```python
from build123d import *

# Parameters (mm, degrees)
SKETCH1_W           = 12
SKETCH1_H           = 4
BOSS_EXTRUDE1_DEPTH = 8
SKETCH2_W           = 4
SKETCH2_H           = 12
BOSS_EXTRUDE2_DEPTH = 25
SKETCH3_W           = 7.5
SKETCH3_H           = 12
BOSS_EXTRUDE3_DEPTH = 4
CHAMFER1_SIZE       = 2
RIB1_REACH          = 35.425
SKETCH4_WALL_W      = 70.36529828
SKETCH4_WALL_H      = 12
RIB2_REACH          = 35.425
SKETCH5_WALL_W      = 70.36529828
SKETCH5_WALL_H      = 12
SKETCH7_R           = 1
CUT_EXTRUDE2_DEPTH  = 4
FILLET1_R           = 0.4


with BuildPart() as part:
    # Sketch1 → Boss-Extrude1 (new body)
    with BuildSketch(Plane(origin=(0, 0, 0), x_dir=(0, 0, -1), z_dir=(1, 0, 0))):
        with Locations((6, 2)):
            Rectangle(SKETCH1_W, SKETCH1_H)
    extrude(amount=BOSS_EXTRUDE1_DEPTH)

    # Sketch2 → Boss-Extrude2 (add)
    with BuildSketch(Plane.XZ):
        with Locations((6, -6)):
            Rectangle(SKETCH2_W, SKETCH2_H)
    extrude(amount=BOSS_EXTRUDE2_DEPTH)

    # Sketch3 → Boss-Extrude3 (add)
    with BuildSketch(Plane.XZ.offset(25)):
        with Locations((7.75, -6)):
            Rectangle(SKETCH3_W, SKETCH3_H)
    extrude(amount=BOSS_EXTRUDE3_DEPTH)

    # Chamfer1
    chamfer1_edges = [part.edges().sort_by_distance(p)[0] for p in [
        (8, 4, -6),
        (4, -29, -6),
    ]]
    chamfer(chamfer1_edges, length=CHAMFER1_SIZE)

    # Sketch4 wall → Rib1 (add, up to next)
    with BuildSketch(Plane(origin=(3.464466094, -0.535533906, -12), x_dir=(0.707106781187, -0.707106781187, 0), z_dir=(-0.707106781187, -0.707106781187, 0)), mode=Mode.PRIVATE) as rib1_sk1:
        with Locations((0, 6)):
            Rectangle(SKETCH4_WALL_W, SKETCH4_WALL_H)
    rib1_tool1 = extrude(rib1_sk1.sketch, amount=-RIB1_REACH, mode=Mode.PRIVATE) - part.part
    add(rib1_tool1.solids().sort_by_distance((3.464466094, -0.535533906, -12))[0])

    # Sketch5 wall → Rib2 (add, up to next)
    with BuildSketch(Plane(origin=(8.535533906, -24.464466094, 0), x_dir=(0.707106781187, -0.707106781187, 0), z_dir=(0.707106781187, 0.707106781187, 0)), mode=Mode.PRIVATE) as rib2_sk1:
        with Locations((0, 6)):
            Rectangle(SKETCH5_WALL_W, SKETCH5_WALL_H)
    rib2_tool1 = extrude(rib2_sk1.sketch, amount=-RIB2_REACH, mode=Mode.PRIVATE) - part.part
    add(rib2_tool1.solids().sort_by_distance((8.535533906, -24.464466094, 0))[0])

    # Sketch7 → Cut-Extrude2 (cut)
    with BuildSketch(Plane.ZY):
        with Locations((-6, 2)):
            Circle(SKETCH7_R)
    extrude(amount=-CUT_EXTRUDE2_DEPTH, mode=Mode.SUBTRACT)

    # Fillet1
    fillet1_edges = [part.edges().sort_by_distance(p)[0] for p in [
        (11.5, -25, -6),
        (11.5, -27, -12),
        (10.285533906, -25, 0),
        (11.5, -27, 0),
        (11.5, -29, -6),
        (8.75, -29, 0),
        (8.75, -29, -12),
        (6, -29, -6),
        (3, 4, -12),
        (4, -14.035533906, -12),
        (7, 3, -12),
        (5, -28, -12),
        (4, -14.035533906, 0),
        (4, -27, -6),
        (8, -10.964466094, 0),
        (3, 4, 0),
        (7, 3, 0),
        (5, -28, 0),
        (0, 4, -6),
        (8, 2, -6),
        (6, 4, -6),
        (0, 2, -12),
        (0, 0, -6),
        (4, -1.071067812, -6),
        (0, 2, 0),
        (1.464466094, 0, -12),
        (1.464466094, 0, 0),
        (3.464466094, -0.535533906, -12),
        (2.928932188, 0, -6),
        (3.464466094, -0.535533906, 0),
        (10.285533906, -25, -12),
        (9.071067812, -25, -6),
        (8, -10.964466094, -12),
        (8.535533906, -24.464466094, 0),
        (8.535533906, -24.464466094, -12),
        (8, -23.928932188, -6),
    ]]
    fillet(fillet1_edges, radius=FILLET1_R)


solid = part.part
```
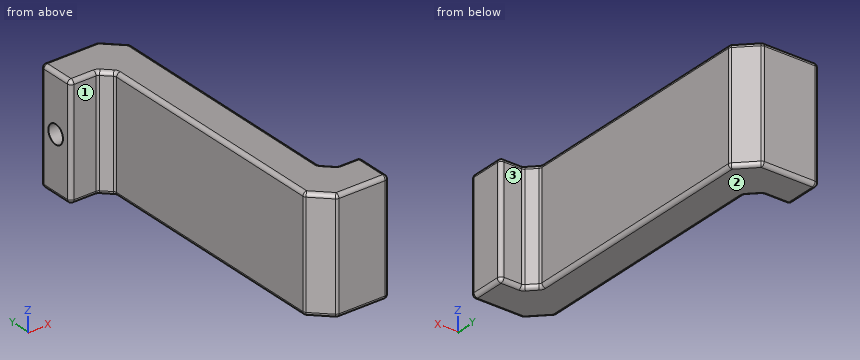
Part model, mm, in its own coordinate system. Face numbers are marked on the shaded views. A direction names the side the tool comes from. Coordinates: 2 decimals unless noted, no trailing zeros. Loops run counter-clockwise (first coordinate to the right, second up) from the corner with the lowest first, then second, coordinate; pieces in that order, holes last. Notation, with made-up numbers: (27.25, 5.5) - (68.25, 5.5) arc R20 cw to (68.25, 21.5) - close; hole circle Ø11 at (83, -0.75). An arc over 180 degrees is marked (long way). Write item = value, one per line. Start each with the question number.
Item 1: Wall check: L1, parallel to Y at x = 1.3, z = -6; L2, parallel to X at y = -22, z = -9; L3, parallel to Y at x = 1.25, z = -3. Give the ranges that are in metal, low to high. Write a range as from..to.
Item 2: Cut at D-D, the plane x = 1. Give the cut face in (y, z), and give its area (3 significant figures).
Item 3: Cut at C-C, the plane y = -3.5. Give the cut face in (x, z).
Item 4: Cut at B-B, the plane z = -0.75. Give the cut face in (x, y), and give its area (3 significant figures).
Item 5: 3-axis set-ups, long thin cutter, end or side, ignore diameter. For the marked faces 1, 2 and 3: which of +Z, -Z, +X, -X, +Y, -Y reach the whole face in a straight line?
Item 6: Flat gauge pins, fed straight in: pin 1 Ø2 at (x, z) = (4.5, -6.5) entering from -Y; pin 2 Ø1.9 at (x, z) = (1.5, -4) entering from -Y; pin 3 Ø1.5 at (x, z) = (10.5, -5) entering from +Y; pin 4 Ø1 at (y, z) = (1.5, -6.5) entering from -X. Where does each tip first touch, or does it go through?
Item 7: Cut at A-A, the plane x = 10.5. Give the cut face in (y, z), and give its area (3 significant figures).
The answers:
q1.L1 = 0..1, 3..4
q1.L2 = 4..8
q1.L3 = 0..4
q2.outline = (0, -11.6) arc R0.4 ccw to (0.4, -12) - (3.6, -12) arc R0.4 ccw to (4, -11.6) - (4, -0.4) arc R0.4 ccw to (3.6, 0) - (0.4, 0) arc R0.4 ccw to (0, -0.4) - close; hole circle Ø2 at (2, -6)
q2.area = 44.7 mm2
q3.outline = (4, -11.6) arc R0.4 ccw to (4.4, -12) - (7.6, -12) arc R0.4 ccw to (8, -11.6) - (8, -0.4) arc R0.4 ccw to (7.6, 0) - (4.4, 0) arc R0.4 ccw to (4, -0.4) - close
q4.outline = (0, 0.4) arc R0.4 ccw to (0.4, 0) - (2.76, 0) arc R0.4 cw to (3.05, -0.12) - (3.88, -0.95) arc R0.4 cw to (4, -1.24) - (4, -26.83) arc R0.4 ccw to (4.12, -27.12) - (5.88, -28.88) arc R0.4 ccw to (6.17, -29) - (11.1, -29) arc R0.4 ccw to (11.5, -28.6) - (11.5, -25.4) arc R0.4 ccw to (11.1, -25) - (9.24, -25) arc R0.4 cw to (8.95, -24.88) - (8.12, -24.05) arc R0.4 cw to (8, -23.76) - (8, 1.83) arc R0.4 ccw to (7.88, 2.12) - (6.12, 3.88) arc R0.4 ccw to (5.83, 4) - (0.4, 4) arc R0.4 ccw to (0, 3.6) - close
q4.area = 159 mm2
q5.face_1 = +Z, -Z, -X, -Y
q5.face_2 = -Z, +X, -X, +Y, -Y
q5.face_3 = +Z, -Z, +X, +Y
q6.pin_1 = -28.5
q6.pin_2 = 0
q6.pin_3 = -25
q6.pin_4 = 0
q7.outline = (-29, -11.6) arc R0.4 ccw to (-28.6, -12) - (-25.4, -12) arc R0.4 ccw to (-25, -11.6) - (-25, -0.4) arc R0.4 ccw to (-25.4, 0) - (-28.6, 0) arc R0.4 ccw to (-29, -0.4) - close
q7.area = 47.9 mm2
